```python
from build123d import *

# Parameters (mm, degrees)
F0_W     = 28.2
F0_H     = 28.2
F1_DEPTH = 32
F2_R     = 11
F3_DEPTH = 2
F5_DEPTH = 18
F7_D     = 2
F7_DEPTH = 4.5
F7_TIP   = 0.600860619
F8_R     = 2


with BuildPart() as f1:
    # F0 (on Front) → F1 (new body)
    with BuildSketch(Plane.XZ):
        Rectangle(F0_W, F0_H)
    extrude(amount=-F1_DEPTH)

    # F2 (on Front) → F3 (join)
    with BuildSketch(Plane.XZ):
        Circle(F2_R)
    extrude(amount=F3_DEPTH)

    # F4 (on face) → F5 (join)
    with BuildSketch(Plane.XZ.offset(2)):
        with BuildLine():
            Line((1.5, 2), (-1.5, 2))
            ThreePointArc((-1.5, 2), (0, -2.5), (1.5, 2))
        make_face()
    extrude(amount=F5_DEPTH)

    # F7
    with Locations(Plane.XZ):
        with Locations((-11.5, 11.5), (11.5, 11.5), (11.5, -11.5), (-11.5, -11.5)):
            Hole(F7_D / 2, depth=F7_DEPTH)
            with Locations((0, 0, -(F7_DEPTH + F7_TIP / 2))):  # 118° drill point
                Cone(0, F7_D / 2, F7_TIP, mode=Mode.SUBTRACT)

    # F8
    f8_edges = [f1.edges().sort_by_distance(p)[0] for p in [
        (14.1, 16, 14.1),
        (14.1, 16, -14.1),
        (-14.1, 16, 14.1),
        (-14.1, 16, -14.1),
    ]]
    fillet(f8_edges, radius=F8_R)


solid = f1.part
```
The model under review builds one solid part; all positions refer to its coordinate system, in mm. A direction names the side the tool comes from. Round coordinates to 2 decimals unless told otherwise and drop trailing zeros. Order: outer loops, then holes, each group sorted by start corner. A loop starts at its lowest first (then second) coordinate and runs counter-clockwise, first axis right, second up.
Item 1: Add section A-A, the plane x = 0. State the section outline as (y, z) points.
Working result:
outline: (-20, -2.5) - (-2, -2.5) - (-2, -11) - (0, -11) - (0, -14.1) - (32, -14.1) - (32, 14.1) - (0, 14.1) - (0, 11) - (-2, 11) - (-2, 2) - (-20, 2) - close
Item 2: Add section C-C, the plane y = -11.5. State the section outline as (x, z) points.
Working result:
outline: (-1.5, 2) arc R2.5 ccw (long way) to (1.5, 2) - close
Item 3: For pin 1 (1.2 mm diameter, centred on x = 11.5, z = 11.5, fed in from -Y); pin 2 (8 mm diameter, centred on x = 1, y = -12, fed in from +Z); pin 3 (1 mm diameter, centred on y = -10.5, z = -1.5, fed in from -X), all flat-tipped, find the tip position at first contact; note any pin that passes through.
Working result:
pin 1: stops at y = 4.74
pin 2: stops at z = 2
pin 3: stops at x = -2.29
Item 4: Draft analysis for pull direction Z (two halves, no side actions). For faces 3 (the flat face through (14.1, 16, 0)), 4 (the conical face through (-11.638, 4.997, 11.394)), 5 (the cylindrical face through (-2.38, -0.99, -10.74)), state which applies: released by +Z, released by -Z, zero draft, split by the parting line, or undercut.
Working result:
face 3: zero draft
face 4: undercut
face 5: split by the parting line
Item 5: Add section D-D, the plane z = 5.25. State the section outline as (x, y) points.
Working result:
outline: (-14.1, 0) - (-9.67, 0) - (-9.67, -2) - (9.67, -2) - (9.67, 0) - (14.1, 0) - (14.1, 32) - (-14.1, 32) - close
Item 6: Add section B-B, the plane z = 0. State the section outline as (x, y) points.
Working result:
outline: (-14.1, 0) - (-11, 0) - (-11, -2) - (-2.5, -2) - (-2.5, -20) - (2.5, -20) - (2.5, -2) - (11, -2) - (11, 0) - (14.1, 0) - (14.1, 32) - (-14.1, 32) - close
Item 7: Machinability: for faces 1 (the cylindrical face through (-10.763, 2.281, -10.824)), 2 (the cylindrical face through (-13.53, 16.22, -13.5)), which of the approach directions +Z, -Z, +X, -X, +Y, -Y give a long, thin tool a straight path to every point of the face, cutting with its end or side? Answer none if there is none.
Working result:
face 1: -Y
face 2: -Z, -X, +Y, -Y
Item 8: To check wall thickness, follow probe 1 along X at (y, z) = (3.6, -11.5); probe 2 along X at (y, z) = (0.5, 11). State the ranges of each line that lie inside material, in increasing order.
Working result:
probe 1: x = -14.1 to -12.5, -10.5 to 10.5, 12.5 to 14.1
probe 2: x = -14.1 to -12.37, -10.63 to 10.63, 12.37 to 14.1
